Check sheet for the modelled part. Datum: model origin and axes. Units: mm. A direction names the side the tool comes from. Give positions to 0.01 mm unless a question says otherwise; leave off trailing zeros. Write each loop counter-clockwise with the first axis right and the second up, starting at its lowest first coordinate (ties: lowest second). Pieces come first, ordered by that corner, then holes. Notation, with made-up numbers: (10.5, 61.25) -> (33.5, 61.25) arc R31 cw to (33.5, 100.25) -> close; hole circle Ø3 at (34.5, -4.5). An arc over 180 degrees is marked (long way). Answer as a JSON object with one key per item and string values.
Autodesk Inventor part; units mm, degrees
ref_plane "YZ Plane" through (0, 0, 0) normal (1, 0, 0) x (0, 1, 0)
ref_plane "XZ Plane" through (0, 0, 0) normal (0, 1, 0) x (-1, 0, 0)
ref_plane "XY Plane" through (0, 0, 0) normal (0, 0, 1) x (1, 0, 0)
sketch "Sketch1" plane through (0, 0, 0) normal (0, 0, 1) x (1, 0, 0)
  line L0 (0, 0) -> (-25.4, 0)
  line L1 (-25.4, 0) -> (-25.4, 25.4)
  line L2 (-25.4, 25.4) -> (0, 25.4)
  line L3 (0, 25.4) -> (0, 0)
  line L4 (-3.175, 22.225) -> (-22.225, 22.225)
  line L5 (-22.225, 22.225) -> (-22.225, 3.175)
  line L6 (-22.225, 3.175) -> (-3.175, 3.175)
  line L7 (-3.175, 3.175) -> (-3.175, 22.225)
  dimension "d2" = 25.4
  dimension "d4" = 25.4
  dimension "d5" = 3.175
extrude "Extrusion1" add sketch "Sketch1" along normal blind 72.39
sketch "Sketch2" plane through (-25.4, 25.4, 0) normal (0, 1, 0) x (1, 0, 0)
  line L0 (0, 0) -> (25.4, 0)
  line L1 (0, 0) -> (0, -72.39)
  line L2 (0, 0) -> (0, -1.905)
  line L3 (12.7, 0) -> (12.7, -1.905)
  line L4 (12.7, -1.905) -> (0, 0)
  line L5 (12.7, -1.905) -> (25.4, 0)
  dimension "d8" = 1.905
  dimension "d9" = 1.905
extrude "Extrusion2" cut sketch "Sketch2" against normal blind 25.4
sketch "Sketch3" plane through (-25.4, 25.4, 72.39) normal (0, 1, 0) x (1, 0, 0)
  line L0 (25.4, 0) -> (0, 0)
  line L1 (25.4, 72.39) -> (25.4, 0)
  line L2 (12.7, 0) -> (12.7, 70.485) construction
  line L3 (12.7, 0) -> (12.7, 6.35)
  circle A0 centre (12.7, 6.35) radius 3.3782
  circle A1 centre (12.7, 19.05) radius 3.3782
  circle A2 centre (12.7, 31.75) radius 3.3782
  circle A3 centre (12.7, 44.45) radius 3.3782
  circle A4 centre (12.7, 57.15) radius 3.3782
  dimension "d12" = 6.35
  dimension "d13" = 6.7564
  dimension "d16" = 12.7
extrude "Extrusion3" cut sketch "Sketch3" against normal blind 25.4
properties part number "V mount" material "Aluminum 6061"
1. Access from +Z, -Z, +X, -X, +Y, -Y to the whole of each face (thin tool, end or side, straight path). Record for faces 4 (the face through (-25.4, 13, 36)), 5 (the face through (-3.175, 13, 36)).
Determined:
{"face 4": "+Z, -Z, -X, +Y, -Y", "face 5": "+Z, -Z"}
2. Sectioned sample at B-B, the plane x = -5. Enter the section's corners in (y, z) (3 decimals).
Determined:
{"outline": "(0, 0.75) -> (3.175, 0.75) -> (3.175, 72.39) -> (0, 72.39) -> close; (22.225, 0.75) -> (25.4, 0.75) -> (25.4, 72.39) -> (22.225, 72.39) -> close"}
3. Scan lines: L1, parallel to Z at x = -12.7, y = 1.25 (3 decimals); L2, parallel to X at y = 17.75, z = 52 (3 decimals); L3, parallel to X at y = 23.75, z = 40.64. Record each from-to range of solid material in increasing order. Write a range as [from, to].
Determined:
{"L1": "[1.905, 11.862], [18.618, 24.562], [31.318, 37.262], [44.018, 49.962], [56.718, 62.662], [69.418, 72.39]", "L2": "[-25.4, -22.225], [-3.175, 0]", "L3": "[-25.4, -16.08], [-9.32, 0]"}
4. Sectioned sample at C-C, the plane y = 17.5. Enter the section's corners in (x, z) (3 decimals), plus the area to 3 significant figures.
Determined:
{"outline": "(-25.4, 0) -> (-22.225, 0.476) -> (-22.225, 72.39) -> (-25.4, 72.39) -> close; (-3.175, 0.476) -> (0, 0) -> (0, 72.39) -> (-3.175, 72.39) -> close", "area": "458 mm^2"}
5. Sectioned sample at D-D, the plane z = 22.5. Enter the section's corners in (x, y) (3 decimals), plus the area to 3 significant figures.
Determined:
{"outline": "(-25.4, 0) -> (0, 0) -> (0, 25.4) -> (-25.4, 25.4) -> close; hole (-22.225, 3.175) -> (-3.175, 3.175) -> (-3.175, 22.225) -> (-22.225, 22.225) -> close", "area": "282 mm^2"}
6. Mould release check, pull along Z, two halves, no side actions. Record for faces 1 (the face through (-2.21, 12.88, 0.33)), 2 (the face through (-13, 25.4, 36)), 3 (the face through (-13.14, 1.61, 11.89)): released by +Z, released by -Z, zero draft, split by the parting line, or undercut.
Determined:
{"face 1": "released by -Z", "face 2": "zero draft", "face 3": "undercut"}
7. Sectioned sample at A-A, the plane z = 66.04. Enter the section's corners in (x, y) (3 decimals), plus the area to 3 significant figures.
Determined:
{"outline": "(-25.4, 0) -> (-16.078, 0) -> (-16.078, 3.175) -> (-22.225, 3.175) -> (-22.225, 22.225) -> (-16.078, 22.225) -> (-16.078, 25.4) -> (-25.4, 25.4) -> close; (-9.322, 0) -> (0, 0) -> (0, 25.4) -> (-9.322, 25.4) -> (-9.322, 22.225) -> (-3.175, 22.225) -> (-3.175, 3.175) -> (-9.322, 3.175) -> close", "area": "239 mm^2"}
